Build history of the part. All positions in model axes, mm. Round coordinates to 2 decimals unless told otherwise and drop trailing zeros. Write each loop counter-clockwise with the first axis right and the second up, starting at its lowest first coordinate (ties: lowest second). Pieces come first, ordered by that corner, then holes. Notation, with made-up numbers: M -8,35.25 L 16,35.25 A14 ccw 16,61.25 Z; hole C -8.5,81 d6. An arc over 180 degrees is marked long. One line per item, written item: value. Start each with the question number.
```python
from build123d import *

# Parameters (mm, degrees)
F0_W     = 76.2
F0_H     = 76.2
F1_DEPTH = 76.2
F2_SIZE  = 25.4
F3_R     = 6.35


with BuildPart() as f1:
    # F0 (on Top) → F1 (new body)
    with BuildSketch(Plane.XY):
        Rectangle(F0_W, F0_H)
    extrude(amount=F1_DEPTH)

    # F2
    f2_edges = [f1.edges().sort_by_distance(p)[0] for p in [
        (0, -38.1, 76.2),
    ]]
    chamfer(f2_edges, length=F2_SIZE)

    # F3
    f3_edges = [f1.edges().sort_by_distance(p)[0] for p in [
        (38.1, 12.7, 76.2),
        (0, 38.1, 76.2),
        (0, -12.7, 76.2),
        (-38.1, 12.7, 76.2),
        (38.1, -38.1, 25.4),
        (38.1, 0, 0),
        (38.1, 38.1, 38.1),
        (0, -38.1, 50.8),
        (38.1, -25.4, 63.5),
        (-38.1, -25.4, 63.5),
        (0, -38.1, 0),
        (-38.1, -38.1, 25.4),
        (-38.1, 0, 0),
        (0, 38.1, 0),
        (-38.1, 38.1, 38.1),
    ]]
    fillet(f3_edges, radius=F3_R)


solid = f1.part
```
Item 1: Drill centre lines: line 1 (Y direction, x = -19.5, z = 6); line 2 (Z direction, x = -32.5, y = -12.5); line 3 (Z direction, x = 29.5, y = -31). Where is each one in solid material? Low to high.
Item 2: Cut at A-A, the plane x = -30. Write the cut outline in (y, z).
Item 3: Drop flat-ended pins along their axis: pin 1 (2 mm diameter, centred on x = -12, y = -27.5, fed in from +Z); pin 2 (5 mm diameter, centred on x = -14, z = 54, fed in from -Y); pin 3 (2 mm diameter, centred on x = 24, y = -23.5, fed in from +Z). Give the stop position or say it passes through.
Computed values:
1. line 1: y = -38.09 to 38.09
1. line 2: z = 0.04 to 75.67
1. line 3: z = 0 to 57.9
2. outline: M -38.1,6.35 A6.35 ccw -31.75,0 L 31.75,0 A6.35 ccw 38.1,6.35 L 38.1,69.85 A6.35 ccw 31.75,76.2 L -10.07,76.2 A6.35 ccw -14.56,74.34 L -36.24,52.66 A6.35 ccw -38.1,48.17 Z
3. pin 1: stops at z = 62.4
3. pin 2: stops at y = -37.16
3. pin 3: stops at z = 66.4
